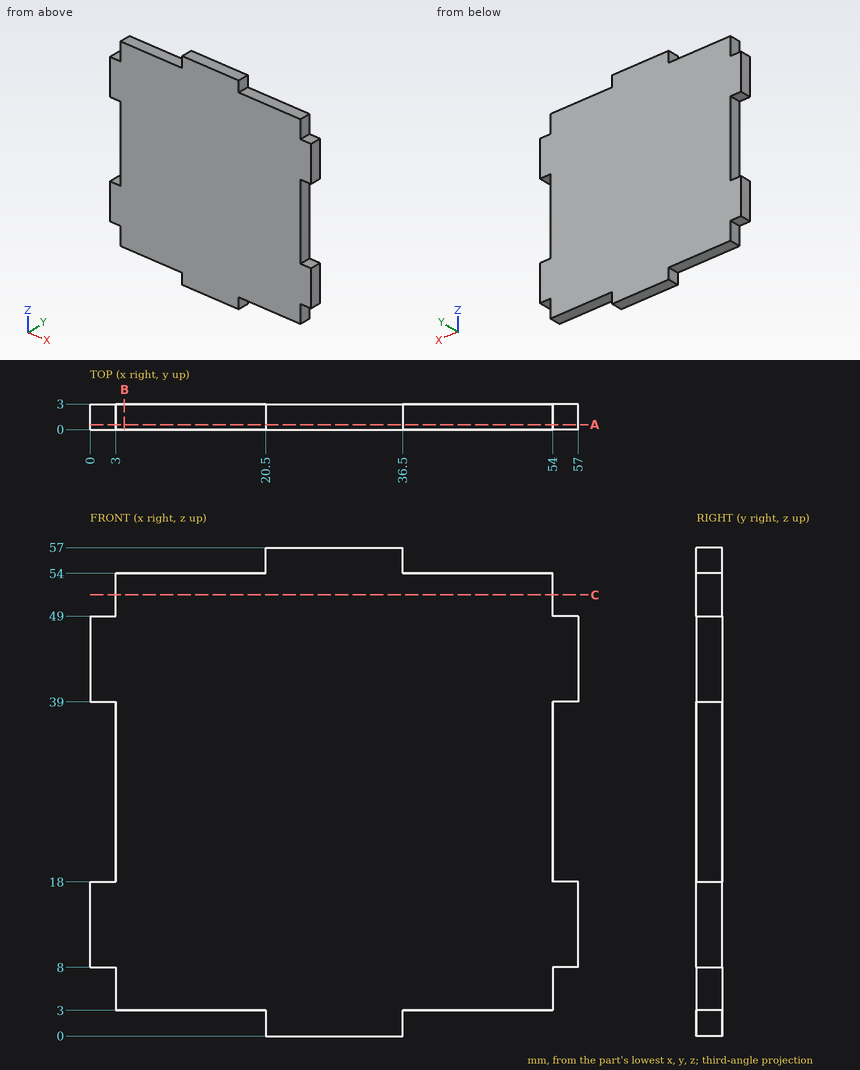
Input: dimensioned drawing with shaded views. Units: mm. Origin: part minimum x, y, z. Round coordinates to 2 decimals unless told otherwise and drop trailing zeros. Loops run counter-clockwise (first coordinate to the right, second up) from the corner with the lowest first, then second, coordinate; pieces in that order, holes last. Notation, with made-up numbers: M 24,24 L 64,24 A17 cw 64,28 Z; hole C -1,82.5 d7. An arc over 180 degrees is marked long. Answer in a Markdown table with one row per item. Add a question column.
1. Section C-C (z = 51.5). Output: boundary loops of the cut face in (x, y), and give its area (3 significant figures).
2. Section B-B (x = 4). Output: boundary loops of the cut face in (y, z), and give its area (3 significant figures).
3. Contact query for flat-ended pins moving along their axis: pin 1 (0.9 mm diameter, centred on x = 55, y = 2, fed in from -Z); pin 2 (1.5 mm diameter, centred on y = 2, z = 5.5, fed in from -X); pin 3 (1.5 mm diameter, centred on x = 55.5, y = 1.5, fed in from +Z). Output: stop coordinate, or through.
4. Section A-A (y = 0.6). Output: boundary loops of the cut face in (x, z), and give its area (3 significant figures).
5. Ray query, probe 1 along Z at (x, y) = (52, 1.2). Return the intervals inside material, ascending.
Values follow:
| question | item | result |
|---|---|---|
| 1 | outline | M 3,0 L 54,0 L 54,3 L 3,3 Z |
| 1 | area | 153 mm^2 |
| 2 | outline | M 0,3 L 3,3 L 3,54 L 0,54 Z |
| 2 | area | 153 mm^2 |
| 3 | pin 1 | z = 8 |
| 3 | pin 2 | x = 3 |
| 3 | pin 3 | z = 49 |
| 4 | outline | M 0,8 L 3,8 L 3,3 L 20.5,3 L 20.5,0 L 36.5,0 L 36.5,3 L 54,3 L 54,8 L 57,8 L 57,18 L 54,18 L 54,39 L 57,39 L 57,49 L 54,49 L 54,54 L 36.5,54 L 36.5,57 L 20.5,57 L 20.5,54 L 3,54 L 3,49 L 0,49 L 0,39 L 3,39 L 3,18 L 0,18 Z |
| 4 | area | 2,820 mm^2 |
| 5 | probe 1 | 3 to 54 |
